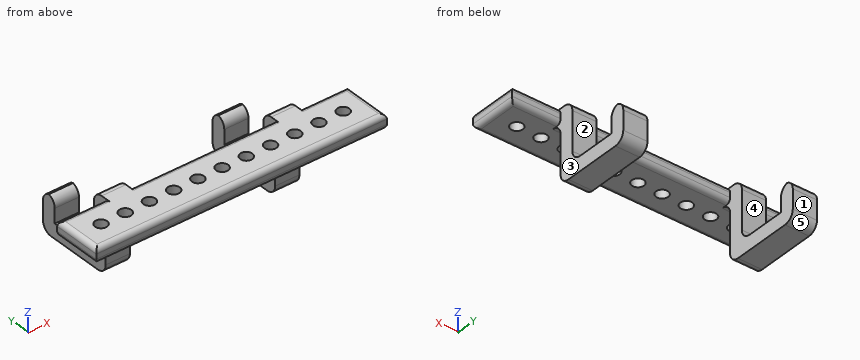
```python
from build123d import *

# Parameters (mm, degrees)
F0_W        = 60
F0_H        = 10
F1_DEPTH    = 3
F2_R        = 1.25
F3_DEPTH    = 3
F4_W        = 5
F4_H        = 15
F5_DEPTH    = 16
F7_DEPTH    = 60
F8_T1_DEPTH = 5
F8_T3_DEPTH = 5
F8_T5_DEPTH = 15
F8_T7_DEPTH = 15
F9_R        = 1


# Not quite as in the source:
# - a fillet or chamfer that OpenCascade refuses, or shapes differently, is made with other operations: its cross-section is extruded or revolved along the edge and cut away or added


with BuildPart() as f1:
    # F0 (on Top) → F1 (new body)
    with BuildSketch(Plane.XY):
        Rectangle(F0_W, F0_H)
    extrude(amount=F1_DEPTH)

    # F2 (on face) → F3 (cut)
    with BuildSketch(Plane.XY.offset(3)):
        with Locations((-25, 0)):
            Circle(F2_R)
        with Locations((-20, 0)):
            Circle(F2_R)
        with Locations((-15, 0)):
            Circle(F2_R)
        with Locations((-10, 0)):
            Circle(F2_R)
        with Locations((-5, 0)):
            Circle(F2_R)
        Circle(F2_R)
        with Locations((5, 0)):
            Circle(F2_R)
        with Locations((10, 0)):
            Circle(F2_R)
        with Locations((15, 0)):
            Circle(F2_R)
        with Locations((20, 0)):
            Circle(F2_R)
        with Locations((25, 0)):
            Circle(F2_R)
    extrude(amount=-F3_DEPTH, mode=Mode.SUBTRACT)

    # F4 (on face) → F5 (join)
    with BuildSketch(Plane(origin=(0, 5, 0), x_dir=(-1, 0, 0), z_dir=(0, 1, 0))):
        with Locations((17.5, -4.5)):
            Rectangle(F4_W, F4_H)
        with Locations((-17.5, -4.5)):
            Rectangle(F4_W, F4_H)
    extrude(amount=F5_DEPTH)

    # F6 (on face) → F7 (cut)
    with BuildSketch(Plane(origin=(-20, 0, 0), x_dir=(0, -1, 0), z_dir=(-1, 0, 0))):
        Polygon((-8, -9), (-8, 3), (-21, 3), (-21, -4), (-18, -4), (-18, -9), align=None)
    extrude(amount=-F7_DEPTH, mode=Mode.SUBTRACT)

    # F8: fillet of radius 2 on 17 edges, made by hand

    # F8_s2 → F8_t1 (join)
    with BuildSketch(Plane.YZ.offset(15)):
        with BuildLine():
            ThreePointArc((3, 0), (4.4142135624, -0.5857864376), (5, -2))
            Line((5, -2), (5, 0))
            Line((5, 0), (3, 0))
        make_face()
        with BuildLine():
            ThreePointArc((10, -9), (8.5857864376, -8.4142135624), (8, -7))
            Line((8, -7), (8, -9))
            Line((8, -9), (10, -9))
        make_face()
    extrude(amount=F8_T1_DEPTH)

    # F8_s4 → F8_t3 (join)
    with BuildSketch(Plane.YZ.offset(-20)):
        with BuildLine():
            ThreePointArc((3, 0), (4.4142135624, -0.5857864376), (5, -2))
            Line((5, -2), (5, 0))
            Line((5, 0), (3, 0))
        make_face()
        with BuildLine():
            ThreePointArc((8, -7), (8.5857864376, -8.4142135624), (10, -9))
            Line((10, -9), (8, -9))
            Line((8, -9), (8, -7))
        make_face()
    extrude(amount=F8_T3_DEPTH)

    # F8_s6 → F8_t5 (cut)
    with BuildSketch(Plane.YZ.offset(-25)):
        with BuildLine():
            ThreePointArc((5, -10), (5.5857864376, -11.4142135624), (7, -12))
            Line((7, -12), (5, -12))
            Line((5, -12), (5, -10))
        make_face()
        with BuildLine():
            ThreePointArc((21, -10), (20.4142135624, -11.4142135624), (19, -12))
            Line((19, -12), (21, -12))
            Line((21, -12), (21, -10))
        make_face()
        with BuildLine():
            ThreePointArc((19, -4), (20.4142135624, -4.5857864376), (21, -6))
            Line((21, -6), (21, -4))
            Line((21, -4), (19, -4))
        make_face()
        with BuildLine():
            ThreePointArc((18, -6), (18.5857864376, -4.5857864376), (20, -4))
            Line((20, -4), (18, -4))
            Line((18, -4), (18, -6))
        make_face()
        with BuildLine():
            ThreePointArc((6, 3), (7.4142135624, 2.4142135624), (8, 1))
            Line((8, 1), (8, 3))
            Line((8, 3), (6, 3))
        make_face()
    extrude(amount=F8_T5_DEPTH, mode=Mode.SUBTRACT)

    # F8_s8 → F8_t7 (cut)
    with BuildSketch(Plane.YZ.offset(10)):
        with BuildLine():
            ThreePointArc((5, -10), (5.5857864376, -11.4142135624), (7, -12))
            Line((7, -12), (5, -12))
            Line((5, -12), (5, -10))
        make_face()
        with BuildLine():
            ThreePointArc((19, -12), (20.4142135624, -11.4142135624), (21, -10))
            Line((21, -10), (21, -12))
            Line((21, -12), (19, -12))
        make_face()
        with BuildLine():
            ThreePointArc((21, -6), (20.4142135624, -4.5857864376), (19, -4))
            Line((19, -4), (21, -4))
            Line((21, -4), (21, -6))
        make_face()
        with BuildLine():
            ThreePointArc((20, -4), (18.5857864376, -4.5857864376), (18, -6))
            Line((18, -6), (18, -4))
            Line((18, -4), (20, -4))
        make_face()
        with BuildLine():
            ThreePointArc((6, 3), (7.4142135624, 2.4142135624), (8, 1))
            Line((8, 1), (8, 3))
            Line((8, 3), (6, 3))
        make_face()
    extrude(amount=F8_T7_DEPTH, mode=Mode.SUBTRACT)

    # F9
    f9_edges = [f1.edges().sort_by_distance(p)[0] for p in [
        (0, -5, 3),
        (30, 0, 3),
        (25, 5, 3),
        (0, 5, 3),
        (-25, 5, 3),
        (-30, 0, 3),
        (0, -5, 0),
        (30, 0, 0),
        (25, 5, 0),
        (0, 5, 0),
        (-25, 5, 0),
        (-30, 0, 0),
    ]]
    fillet(f9_edges, radius=F9_R)


solid = f1.part
```
Geometry check sheet. Reference: the model listing, model coordinates, mm. Face numbers are marked on the shaded views. A direction names the side the tool comes from. Give positions to 0.01 mm unless a question says otherwise; leave off trailing zeros. Loops run counter-clockwise (first coordinate to the right, second up) from the corner with the lowest first, then second, coordinate; pieces in that order, holes last. Notation, with made-up numbers: M 13.25,-34.5 L 65.25,-34.5 A16 ccw 65.25,-12.5 Z; hole C 7.25,-12 d4. An arc over 180 degrees is marked long. Write item = value, one per line.
(1) Gauge pin test, flat ends, axial feed: pin 1 Ø1 at (x, y) = (-23, 5) entering from -Z; pin 2 Ø1.5 at (x, y) = (-20, 0) entering from +Z; pin 3 Ø6.5 at (x, y) = (2.5, -1.5) entering from -Z; pin 4 Ø5.5 at (x, z) = (-16.5, -1.5) entering from +Y. Record the tip position at first contact, or that the pin passes through.
Answer below:
pin_1 = 0.13
pin_2 = through
pin_3 = 0
pin_4 = 19.97
(2) Release check for a two-part mould opening along Y. For the marked faces 3, 4 and 5 record: released by +Y, released by -Y, zero draft, split by the parting line, or undercut.
Answer below:
face_3 = zero draft
face_4 = undercut
face_5 = released by +Y
(3) Sectioned sample at D-D, the plane z = -1. Record the cut outline in (x, y), plus the area to 3 significant figures.
Answer below:
outline = M -20,4.73 L -15,4.73 L -15,8 L -20,8 Z; M 15,4.73 L 20,4.73 L 20,8 L 15,8 Z
area = 32.7 mm2
(4) Tool access check on the marked faces 1 and 2. Record the directions out of +Z, -Z, +X, -X, +Y, -Y that give a thin tool (end or side, any length) a straight path to the whole face; none if there is none.
Answer below:
face_1 = +Z, -Z, +X, -X, +Y
face_2 = +Z, +X, -X
(5) Sectioned sample at A-A, the plane x = 5. Record the cut outline in (y, z).
Answer below:
outline = M -5,1 A1 ccw -4,0 L -1.25,0 L -1.25,3 L -4,3 A1 ccw -5,2 Z; M 1.25,0 L 4,0 A1 ccw 5,1 L 5,2 A1 ccw 4,3 L 1.25,3 Z
(6) Material ranges on line 1 (Y direction, x = 25, z = 1.45); line 2 (Z direction, x = 3.5, y = -3.5); line 3 (Y direction, x = -17, z = -2.5), recorded low to high. Write a range as [from, to].
Answer below:
line_1 = [-5, -1.25], [1.25, 5]
line_2 = [0, 3]
line_3 = [5, 8]
(7) Sectioned sample at C-C, the plane z = -8.25. Record the cut outline in (x, y).
Answer below:
outline = M -20,5 L -15,5 L -15,8.44 L -20,8.44 Z; M -20,18 L -15,18 L -15,21 L -20,21 Z; M 15,5 L 20,5 L 20,8.44 L 15,8.44 Z; M 15,18 L 20,18 L 20,21 L 15,21 Z
(8) Sectioned sample at B-B, the plane y = 10.75. Record the cut outline in (x, z), plus the area to 3 significant figures.
Answer below:
outline = M -20,-12 L -15,-12 L -15,-9 L -20,-9 Z; M 15,-12 L 20,-12 L 20,-9 L 15,-9 Z
area = 30.0 mm2
